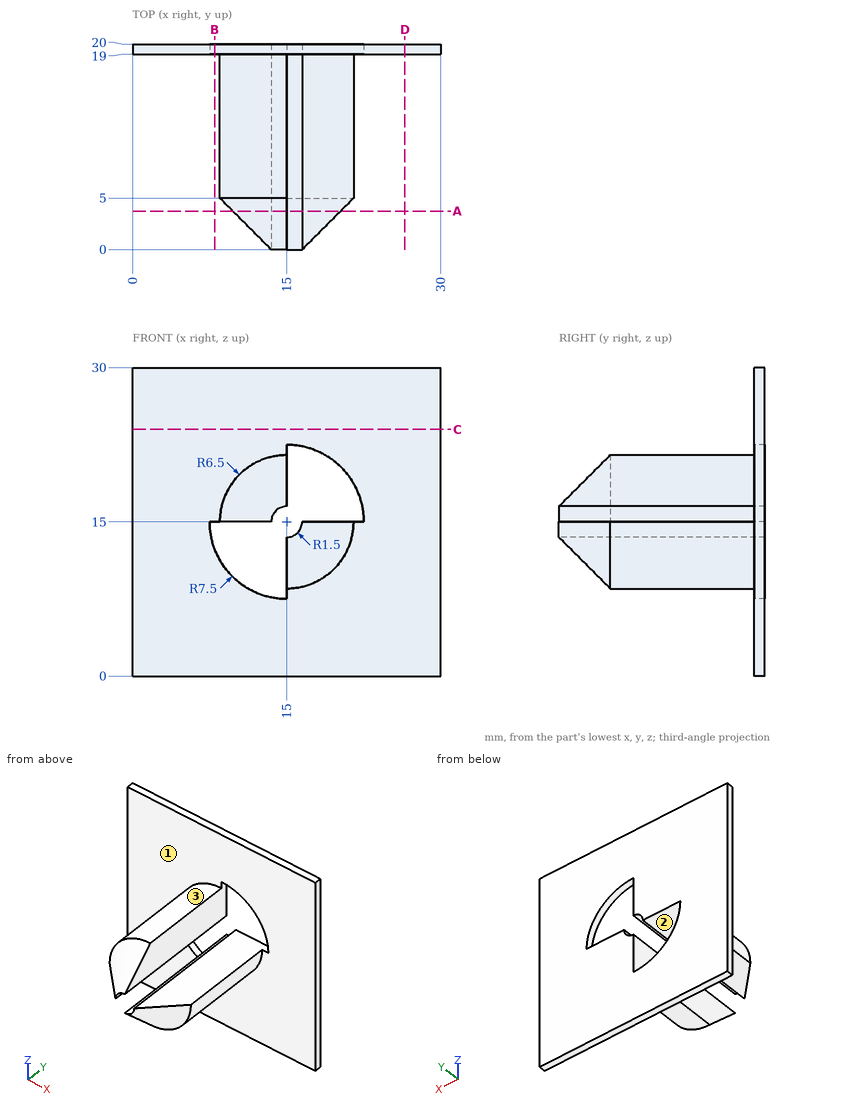
Drawing for the job (mm, zero at the part's lowest x, y, z). A direction names the side the tool comes from. Give positions to 0.01 mm unless a question says otherwise; leave off trailing zeros. Order: outer loops, then holes, each group sorted by start corner. A loop starts at its lowest first (then second) coordinate and runs counter-clockwise, first axis right, second up. Notation, with made-up numbers: M -34,-4.75 L 25,-4.75 A26 cw 25,15.25 Z; hole C -28,5.25 d9. An arc over 180 degrees is marked long. Put each result on its own line as item: value. Start each with the question number.
(1) Drill centre lines: line 1 along Y through (x, z) = (4, 24); line 2 along X through (y, z) = (16, 14); line 3 along Y through (x, z) = (16.75, 9). Where is each one in solid material? Low to high.
(2) Saw through at A-A, the plane y = 3.75. Write the cut outline in (x, z).
(3) Saw through at C-C, the plane z = 24. Write the cut outline in (x, y), then the cut area to 3 significant figures.
(4) Flat gauge pins, fed straight in: pin 1 Ø1.5 at (y, z) = (4, 13.5) entering from +X; pin 2 Ø1.8 at (y, z) = (10, 18) entering from +X; pin 3 Ø5 at (x, y) = (20.5, 14.5) entering from -Z. Where does each tip first touch, or does it go through?
(5) Which spindle directions (+Z, -Z, +X, -X, +Y, -Y) get a long thin tool onto all of the face, cutting with end or side? Do the marked faces 1, 2 and 3. Say none if no direction does.
(6) Saw through at B-B, the plane x = 8. Write the cut outline in (y, z).
(7) Saw through at D-D, the plane x = 26.5. Write the cut outline in (y, z), then the cut area to 3 significant figures.
Check result:
1. line 1: y = 19 to 20
1. line 2: x = 16.12 to 21.42
1. line 3: y = 4.75 to 20
2. outline: M 9.75,15 L 13.5,15 A1.5 cw 15,16.5 L 15,20.25 A5.25 ccw Z; M 15,9.75 A5.25 ccw 20.25,15 L 16.5,15 A1.5 cw 15,13.5 Z
3. outline: M 0,19 L 30,19 L 30,20 L 0,20 Z
3. area: 30.0 mm2
4. pin 1: stops at x = 21.09
4. pin 2: stops at x = 15
4. pin 3: stops at z = 9.23
5. face 1: -Y
5. face 2: +Y, -Y
5. face 3: +Z, -X, -Y
6. outline: M 19,0 L 20,0 L 20,12.31 L 19,12.31 Z; M 19,15 L 20,15 L 20,30 L 19,30 Z
7. outline: M 19,0 L 20,0 L 20,30 L 19,30 Z
7. area: 30.0 mm2
